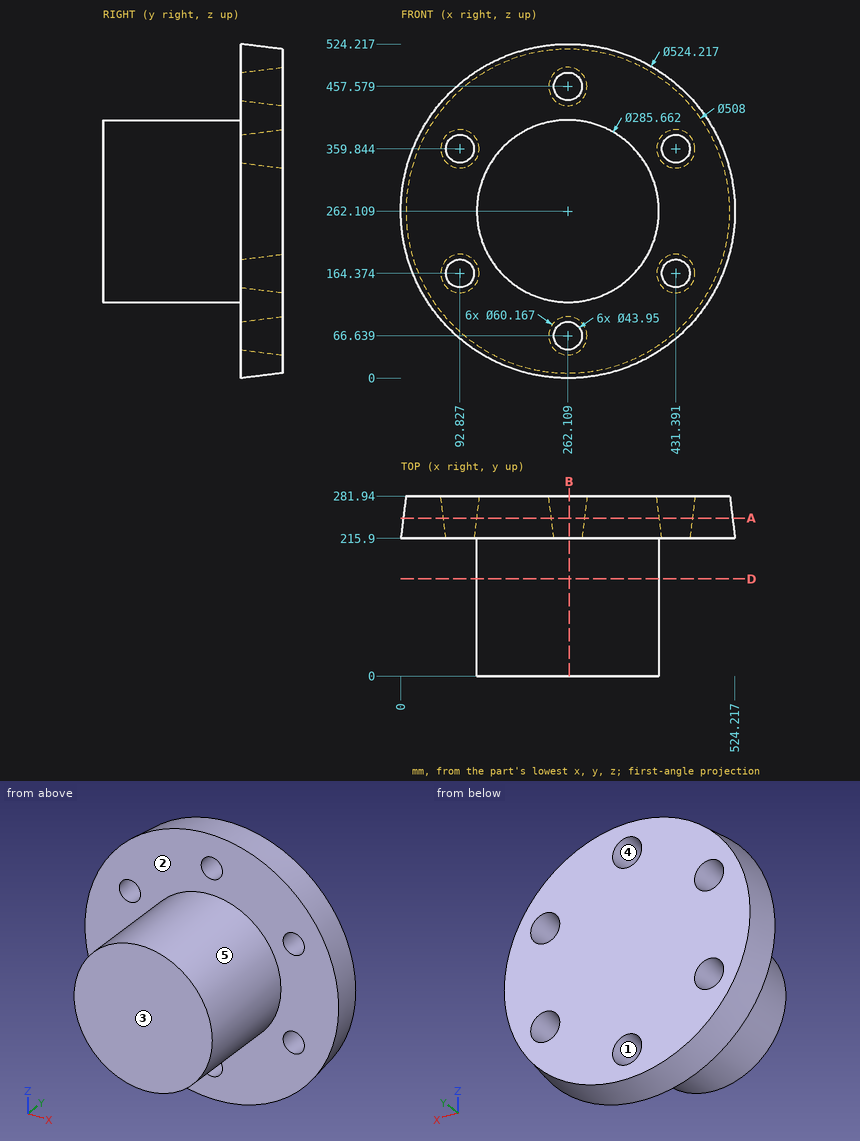
Can you work these out from the drawing? Everything is in mm from the part's minimum corner. A direction names the side the tool comes from. Round coordinates to 2 decimals unless told otherwise and drop trailing zeros. Write each loop counter-clockwise with the first axis right and the second up, starting at its lowest first coordinate (ties: lowest second). Pieces come first, ordered by that corner, then holes.
1. Suppose I cut it at A-A (y = 247.5). List the corners of the cut face in (x, z) for me (1 decimal).
2. Will these pins go through, and if not, where does the flat tip stop? pin 1 Ø1.5 at (x, y) = (397.5, 229.5) entering from +Z; pin 2 Ø6 at (y, z) = (229, 413.5) entering from +X; pin 3 Ø5 at (x, y) = (238, 83.5) entering from +Z.
3. I need wall thicknesses on L1, parallel to Y at x = 112, z = 137; L2, parallel to X at y = 264, z = 70.5 (1 decimal); L3, parallel to X at y = 222, z = 476 (1 decimal). Which ranges of each line are inside material? Lowest first, please.
4. Suppose I cut it at D-D (y = 152.5). List the corners of the cut face in (x, z) for me.
5. Suppose I cut it at B-B (x = 264). State how many separate pieces and enclosed holes the cut face has, and give its area (3 significant figures).
6. For the marked faces 1 and 2, which set-ups out of +Z, -Z, +X, -X, +Y, -Y let a thin tool reach every point of the face, with its end or its side?
7. If we mould it in two halves opening along X, with no side actions, what happens to the marked faces 3, 4 and 5? For each: released by +X, released by -X, zero draft, split by the parting line, or undercut.
Answer sheet:
1. outline: circle Ø516.5 at (262.1, 262.1); hole circle Ø51.7 at (92.8, 164.4); hole circle Ø51.7 at (92.8, 359.8); hole circle Ø51.7 at (262.1, 66.6); hole circle Ø51.7 at (262.1, 457.6); hole circle Ø51.7 at (431.4, 164.4); hole circle Ø51.7 at (431.4, 359.8)
2. pin 1: stops at z = 485.06
2. pin 2: stops at x = 476.26
2. pin 3: stops at z = 403.3
3. L1: y = 215.9 to 281.94
3. L2: x = 92 to 234.5, 289.7 to 432.2
3. L3: x = 111.9 to 248.8, 275.4 to 412.3
4. outline: circle Ø285.66 at (262.11, 262.11)
5. separate pieces: 3
5. enclosed holes: 0
5. area: 88,900 mm2
6. face 1: +Y
6. face 2: -Y
7. face 3: zero draft
7. face 4: undercut
7. face 5: split by the parting line
